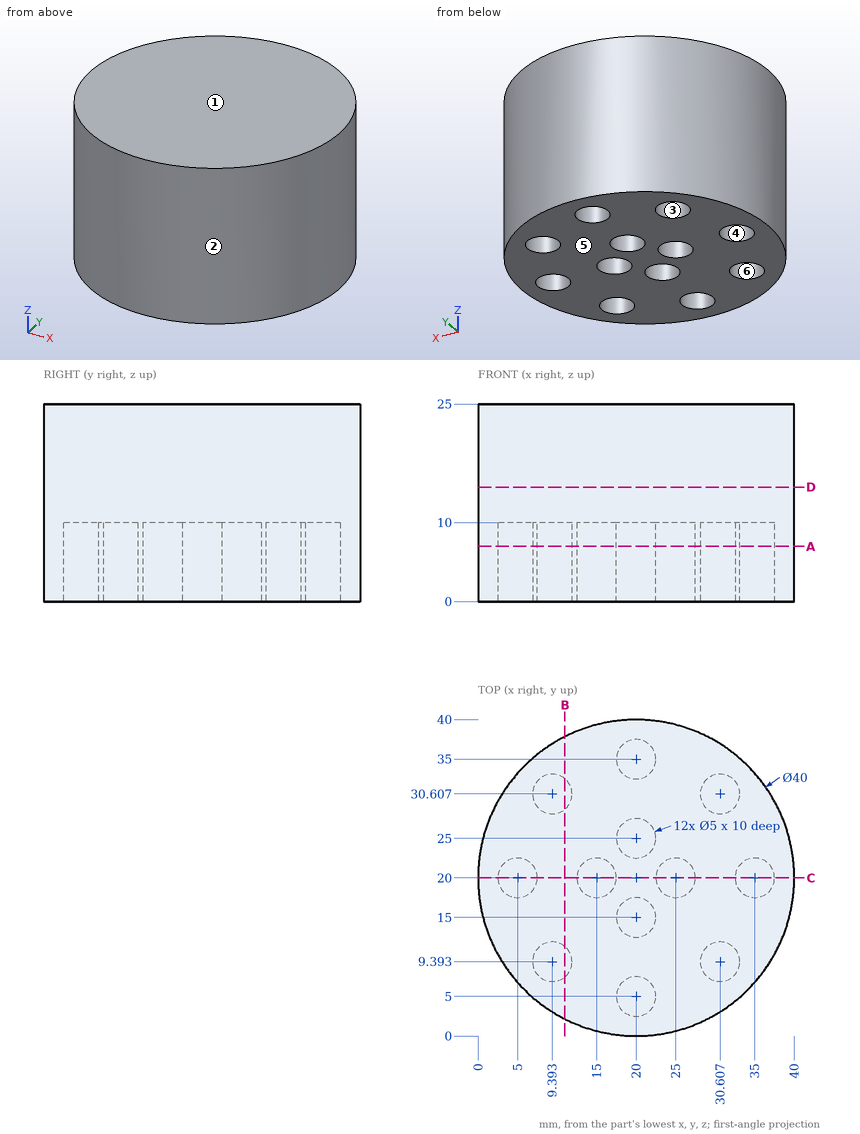
Study the drawing (mm; zero at the part's minimum x, y, z) and answer. A direction names the side the tool comes from. Give positions to 0.01 mm unless a question says otherwise; leave off trailing zeros. Order: outer loops, then holes, each group sorted by start corner. A loop starts at its lowest first (then second) coordinate and runs counter-clockwise, first axis right, second up.
1) Find section D-D on z = 14.5. Write down the section's boundary in (x, y), then the cut area to 3 significant figures.
Reported:
outline: circle Ø40 at (20, 20)
area: 1,260 mm2
2) Find section B-B on x = 11. Write down the section's boundary in (y, z).
Reported:
outline: (2.14, 0) - (7.48, 0) - (7.48, 10) - (11.31, 10) - (11.31, 0) - (28.69, 0) - (28.69, 10) - (32.52, 10) - (32.52, 0) - (37.86, 0) - (37.86, 25) - (2.14, 25) - close
3) For the marked faces 5 and 6, determine the directions among +Z, -Z, +X, -X, +Y, -Y from which every point of the face is accessible in a straight line to the end or side of a thin tool.
Reported:
face 5: -Z, +X, -X, +Y, -Y
face 6: -Z
4) Find section C-C on y = 20. Write down the section's boundary in (x, z), then the cut area to 3 significant figures.
Reported:
outline: (0, 0) - (2.5, 0) - (2.5, 10) - (7.5, 10) - (7.5, 0) - (12.5, 0) - (12.5, 10) - (17.5, 10) - (17.5, 0) - (22.5, 0) - (22.5, 10) - (27.5, 10) - (27.5, 0) - (32.5, 0) - (32.5, 10) - (37.5, 10) - (37.5, 0) - (40, 0) - (40, 25) - (0, 25) - close
area: 800 mm2
5) Determine the mould class of the marked faces 1, 2, 3 and 4 for opening direction X: pulls with the +X half, pulls with the -X half, needs draft (parallel to the pull), parting line crosses it, or undercut.
Reported:
face 1: needs draft
face 2: parting line crosses it
face 3: undercut
face 4: undercut
6) Given P1, Ø4.5, axis at x = 15, y = 20, coming from the -Z side; P2, Ø3, axis at y = 4.5, z = 14, coming from the +X side; P3, Ø5, axis at y = 34, z = 16, coming from the -X side, each flat-ended and moving along its own axis, determine where each tip first touches the part or whether it passes through.
Reported:
P1: stops at z = 10
P2: stops at x = 34.28
P3: stops at x = 3.64
7) Find section A-A on z = 7. Give the number of separate pieces and of enclosed holes in the cut face, then the cut area to 3 significant figures.
Reported:
separate pieces: 1
enclosed holes: 12
area: 1,020 mm2
8) Consider line 1 along Y through (x, z) = (20, 3.5); line 2 along X through (y, z) = (18.5, 3) (1 decimal); line 3 along X through (y, z) = (31, 5) (1 decimal). Determine where each line is inside the solid, lowest interval first.
Reported:
line 1: y = 0 to 2.5, 7.5 to 12.5, 17.5 to 22.5, 27.5 to 32.5, 37.5 to 40
line 2: x = 0.1 to 3, 7 to 13, 17 to 23, 27 to 33, 37 to 39.9
line 3: x = 3.3 to 6.9, 11.9 to 28.1, 33.1 to 36.7
